from build123d import *

# Parameters (mm, degrees)
SKETCH1_R           = 0.75
BOSS_EXTRUDE4_DEPTH = 1.5
SKETCH1_6_R         = 1.5
BOSS_EXTRUDE5_DEPTH = 2.5
BOSS_EXTRUDE6_START = 1.5
SKETCH1_7_R         = 1
BOSS_EXTRUDE6_DEPTH = 2.4
SWEEP2_PITCH        = 1
BOSS_EXTRUDE7_START = 3.9
SKETCH1_8_R         = 0.75
BOSS_EXTRUDE7_DEPTH = 1.5
CUT_EXTRUDE2_START  = -1
CUT_EXTRUDE2_DEPTH  = 1
FILLET2_R           = 0.1


with BuildPart() as part:
    # Sketch1 → Boss-Extrude4 (new body)
    with BuildSketch(Plane(origin=(0, 0, 0), x_dir=(0, 0, -1), z_dir=(1, 0, 0))):
        Circle(SKETCH1_R)
    extrude(amount=BOSS_EXTRUDE4_DEPTH)

    # Sketch1<6> → Boss-Extrude5 (add)
    with BuildSketch(Plane(origin=(0, 0, 0), x_dir=(0, 0, -1), z_dir=(1, 0, 0))):
        Circle(SKETCH1_6_R)
    extrude(amount=-BOSS_EXTRUDE5_DEPTH)

    # Sketch1<7> → Boss-Extrude6 (add)
    with BuildSketch(Plane(origin=(0, 0, 0), x_dir=(0, 0, -1), z_dir=(1, 0, 0)).offset(BOSS_EXTRUDE6_START)):
        Circle(SKETCH1_7_R)
    extrude(amount=BOSS_EXTRUDE6_DEPTH)

    # Sweep2: the profile of Sketch7 profile screwed along a right-hand helix of 2 turns, 8 arcs to a turn; built about Z, then put on its axis
    sweep2_z = Axis((0, 0, 0), (0, 0, 1))
    sweep2_corners = [(1.5003, 0, -0.25), (1.5003, 0, 0.15), (1, 0, 0.15), (1, 0, -0.25)]
    with BuildLine(mode=Mode.PRIVATE) as sweep2_profile:
        Line(sweep2_corners[0], sweep2_corners[1])
        Line(sweep2_corners[1], sweep2_corners[2])
        Line(sweep2_corners[2], sweep2_corners[3])
        Line(sweep2_corners[3], sweep2_corners[0])
    sweep2_cap = Face(sweep2_profile.wire())
    sweep2_turn_angles = [0, 22.5, 45, 67.5, 90, 112.5, 135, 157.5, 180, 202.5, 225, 247.5, 270, 292.5, 315, 337.5, 360]
    sweep2_turn_weights = [1, 0.9238795325112867, 1, 0.9238795325112867, 1, 0.9238795325112867, 1, 0.9238795325112867, 1, 0.9238795325112867, 1, 0.9238795325112867, 1, 0.9238795325112867, 1, 0.9238795325112867, 1]
    sweep2_turn_rails = [Edge.make_bspline([Vector(p[0], p[1], 0).rotate(sweep2_z, sweep2_turn_angles[k]) / sweep2_turn_weights[k] + Vector(0, 0, p[2] + SWEEP2_PITCH * sweep2_turn_angles[k] / 360) for k in range(17)], [0, 0, 0, 1, 1, 2, 2, 3, 3, 4, 4, 5, 5, 6, 6, 7, 7, 8, 8, 8], 2, sweep2_turn_weights) for p in sweep2_corners]
    sweep2_turn_sides = [Face.make_surface_from_curves(sweep2_turn_rails[p[0]], sweep2_turn_rails[p[1]]) for p in [(0, 1), (1, 2), (2, 3), (3, 0)]]
    sweep2 = Plane(origin=(1.75, 0, 0), x_dir=(0, 0, -1), z_dir=(1, 0, 0)) * Solid(Shell([*[p.moved(Location((0, 0, SWEEP2_PITCH * i))) for i in range(2) for p in sweep2_turn_sides], sweep2_cap, sweep2_cap.rotate(sweep2_z, 720).moved(Location((0, 0, SWEEP2_PITCH * 720 / 360)))]))
    add(sweep2)

    # Sketch1<8> → Boss-Extrude7 (add)
    with BuildSketch(Plane(origin=(0, 0, 0), x_dir=(0, 0, -1), z_dir=(1, 0, 0)).offset(BOSS_EXTRUDE7_START)):
        Circle(SKETCH1_8_R)
    extrude(amount=BOSS_EXTRUDE7_DEPTH)

    # Sketch8 → Cut-Extrude2 (cut)
    with BuildSketch(Plane.ZY.offset(2.5).offset(CUT_EXTRUDE2_START)):
        with BuildLine():
            Line((0.3, 1.469693846), (0.3, 0.3))
            Line((0.3, 0.3), (1.469693846, 0.3))
            ThreePointArc((1.469693846, 0.3), (1.5, 0), (1.469693846, -0.3))
            Line((1.469693846, -0.3), (0.3, -0.3))
            Line((0.3, -0.3), (0.3, -1.469693846))
            ThreePointArc((0.3, -1.469693846), (0, -1.5), (-0.3, -1.469693846))
            Line((-0.3, -1.469693846), (-0.3, -0.3))
            Line((-0.3, -0.3), (-1.469693846, -0.3))
            ThreePointArc((-1.469693846, -0.3), (-1.5, 0), (-1.469693846, 0.3))
            Line((-1.469693846, 0.3), (-0.3, 0.3))
            Line((-0.3, 0.3), (-0.3, 1.469693846))
            ThreePointArc((-0.3, 1.469693846), (0, 1.5), (0.3, 1.469693846))
        make_face()
    extrude(amount=CUT_EXTRUDE2_DEPTH, mode=Mode.SUBTRACT)

    # Sketch9 → Revolve2 (revolve)
    with BuildSketch(Plane(origin=(0, 0, 0), x_dir=(1, 0, 0), z_dir=(0, 1, 0)), mode=Mode.PRIVATE) as revolve2_sk:
        Polygon((5.4, 0), (5.4, 1), (6.9, 0.5), (6.9, 0), align=None)
    revolve(revolve2_sk.sketch.rotate(Axis((0, 0, 0), (1, 0, 0)), 180), axis=Axis((0, 0, 0), (1, 0, 0)))

    # Fillet2
    fillet2_edges = [part.edges().sort_by_distance(p)[0] for p in [
        (5.4, 0, -1),
    ]]
    fillet(fillet2_edges, radius=FILLET2_R)


solid = part.part
Geometry: final body of the model. Coordinates: model frame, mm. A direction names the side the tool comes from. Round coordinates to 2 decimals unless told otherwise and drop trailing zeros. Loops run counter-clockwise (first coordinate to the right, second up) from the corner with the lowest first, then second, coordinate; pieces in that order, holes last. Notation, with made-up numbers: M 26.5,47 L 70.5,47 A19 cw 70.5,61 Z; hole C -2.5,83.25 d10. An arc over 180 degrees is marked long. Put each result on its own line as item: value. Start each with the question number.
(1) Material intervals for line 1 along X through (y, z) = (1.1, -0.6); line 2 along X through (y, z) = (0.6, 1); line 3 along Y through (x, z) = (-1.75, 1.35), sorted ascending. Write a range as [from, to].
(2) Section query B-B (x = 4.25). Return loops of the section in (y, z).
(3) Section query C-C (y = -1.1). State how many separate pieces and enclosed holes the cut face has, then the cut area to 3 significant figures.
(4) Set-up query: faces 1 (the face through (4.64, 0.03, 0.75)), 2 (the face through (-2, 0.3, 1)), 3 (the face through (-2, 1, -0.3)). Return all of +Z, -Z, +X, -X, +Y, -Y with unobstructed straight access to the full face (end or side cutting, diameter ignored); none if empty.
(5) Draft query along Y for faces 4 (the face through (-1.232, -0.575, -1.386)), 5 (the face through (-2, -0.3, -1)), 6 (the face through (-2, 1, 0.3)). Return one class per face: +Y half, -Y half, draft (parallel to the pull), parting line (faces both ways), or undercut.
(6) Section query A-A (x = -2). Return loops of the section in (y, z).
(7) Contact query for flat-ended pins moving along their axis: pin 1 Ø0.5 at (x, y) = (-2, 1) entering from -Z; pin 2 Ø0.8 at (x, z) = (-2, 1) entering from +Y; pin 3 Ø0.8 at (x, y) = (-2, -1) entering from -Z. Output: stop coordinate, or through.
Findings below:
1. line 1: x = [-2.5, 0], [1.67, 2.07], [2.67, 3.07]
1. line 2: x = [-2.5, 0], [1.91, 2.31], [2.91, 3.31]
1. line 3: y = [-0.65, -0.3], [0.3, 0.65]
2. outline: C 0,0 d1.5
3. separate pieces: 3
3. enclosed holes: 0
3. area: 6.13 mm2
4. face 1: none
4. face 2: +Z, -Z, -X
4. face 3: -X, +Y, -Y
5. face 4: parting line
5. face 5: undercut
5. face 6: draft
6. outline: M -1.47,-0.3 A1.5 ccw -0.3,-1.47 L -0.3,-0.3 Z; M -1.47,0.3 L -0.3,0.3 L -0.3,1.47 A1.5 ccw Z; M 0.3,-1.47 A1.5 ccw 1.47,-0.3 L 0.3,-0.3 Z; M 0.3,0.3 L 1.47,0.3 A1.5 ccw 0.3,1.47 Z
7. pin 1: stops at z = -1.3
7. pin 2: stops at y = 1.37
7. pin 3: stops at z = -1.37
